Design review of the part built by this model. Coordinates are the model's own, in mm. Face numbers are marked on the shaded views. A direction names the side the tool comes from. Give positions to 0.01 mm unless a question says otherwise; leave off trailing zeros. Loops run counter-clockwise (first coordinate to the right, second up) from the corner with the lowest first, then second, coordinate; pieces in that order, holes last. Notation, with made-up numbers: (66, 23) -> (95, 23) arc R34 ccw to (95, 57) -> close; hole circle Ø8 at (45, 44). An arc over 180 degrees is marked (long way). Use a Markdown table: item, result. Add a question column.
1. Add section B-B (y = 27). State the section outline as (x, z) points, and give its area (4 significant figures).
2. Add section C-C (x = 7). State the section outline as (y, z) points, and give its area (3 significant figures).
3. Add section A-A (z = 5). State the section outline as (x, y) points.
4. For the marked faces 1 and 2, list the 3-axis set-ups (+Z, -Z, +X, -X, +Y, -Y) from which the entire face can be reached by the end or side of a thin tool; tool diameter is ignored.
5. To check wall thickness, follow line 1 (X direction, y = 59, z = 18.5); line 2 (Y direction, x = 26.5, z = 19.25). State the ranges of each line that lie inside material, in increasing order.
6. Draft analysis for pull direction X (two halves, no side actions). For the marked faces 3, 4, 5 and 6, state which applies: pulls with the +X half, pulls with the -X half, needs draft (parallel to the pull), parting line crosses it, or undercut.
7. For pin 1 Ø8 at (x, z) = (72.5, 22.5) entering from -Y, flat-tipped, find the tip position at first contact; note if it passes through.
```python
from build123d import *

# Parameters (mm, degrees)
F0_W     = 110
F0_H     = 110
F0_W_2   = 106
F0_H_2   = 106
F1_DEPTH = 25
F2_W     = 106
F2_H     = 106
F3_DEPTH = 1.5
F4_W     = 25
F4_H     = 25
F5_DEPTH = 25
F6_R     = 26.255837
F7_DEPTH = 1.5
F9_DEPTH = 25


with BuildPart() as f1:
    # F0 (on Top) → F1 (new body)
    with BuildSketch(Plane.XY):
        with Locations((55, 55)):
            Rectangle(F0_W, F0_H)
        with Locations((55, 55)):
            Rectangle(F0_W_2, F0_H_2, mode=Mode.SUBTRACT)
    extrude(amount=F1_DEPTH)

    # F2 (on Top) → F3 (join)
    with BuildSketch(Plane.XY):
        with Locations((55, 55)):
            Rectangle(F2_W, F2_H)
    extrude(amount=F3_DEPTH)

    # F4 (on Top) → F5 (cut)
    with BuildSketch(Plane.XY):
        with Locations((23.550745, 87.610851)):
            Rectangle(F4_W, F4_H)
        with Locations((23.550745, 55.610851)):
            Rectangle(F4_W, F4_H)
        with Locations((23.550745, 23.610851)):
            Rectangle(F4_W, F4_H)
        with Locations((55.550745, 87.610851)):
            Rectangle(F4_W, F4_H)
        with Locations((55.550745, 55.610851)):
            Rectangle(F4_W, F4_H)
        with Locations((55.550745, 23.610851)):
            Rectangle(F4_W, F4_H)
        with Locations((87.550745, 87.610851)):
            Rectangle(F4_W, F4_H)
        with Locations((87.550745, 55.610851)):
            Rectangle(F4_W, F4_H)
        with Locations((87.550745, 23.610851)):
            Rectangle(F4_W, F4_H)
    extrude(amount=F5_DEPTH, mode=Mode.SUBTRACT)

    # F6 (on face) → F7 (join, through all)
    with BuildSketch(Plane.XY.offset(1.5)):
        with Locations((55.742927, 79.293631)):
            Circle(F6_R)
    extrude(amount=-F7_DEPTH)

    # F8 (on face) → F9 (cut)
    with BuildSketch(Plane.XZ):
        with BuildLine():
            Line((100.912742, 28.472882), (10.870284, 28.621467))
            ThreePointArc((10.870284, 28.621467), (55.864304, 12.058173), (100.912742, 28.472882))
        make_face()
    extrude(amount=-F9_DEPTH, mode=Mode.SUBTRACT)


solid = f1.part
```
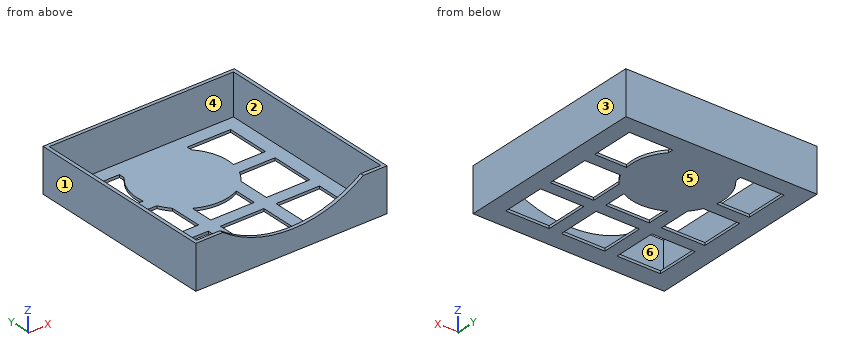
Taken from the geometry:
| question | item | result |
|---|---|---|
| 1 | outline | (0, 0) -> (11.05, 0) -> (11.05, 1.5) -> (2, 1.5) -> (2, 25) -> (0, 25) -> close; (36.05, 0) -> (43.05, 0) -> (43.05, 1.5) -> (36.05, 1.5) -> close; (68.05, 0) -> (75.05, 0) -> (75.05, 1.5) -> (68.05, 1.5) -> close; (100.05, 0) -> (110, 0) -> (110, 25) -> (108, 25) -> (108, 1.5) -> (100.05, 1.5) -> close |
| 1 | area | 146.5 mm^2 |
| 2 | outline | (0, 0) -> (110, 0) -> (110, 25) -> (108, 25) -> (108, 1.5) -> (2, 1.5) -> (2, 25) -> (0, 25) -> close |
| 2 | area | 259 mm^2 |
| 3 | outline | (0, 0) -> (110, 0) -> (110, 110) -> (0, 110) -> close; hole (2, 2) -> (108, 2) -> (108, 108) -> (2, 108) -> close |
| 4 | face 1 | +Z, -Z, -X, +Y, -Y |
| 4 | face 2 | +Z |
| 5 | line 1 | x = 0 to 2, 108 to 110 |
| 5 | line 2 | y = 108 to 110 |
| 6 | face 3 | pulls with the +X half |
| 6 | face 4 | undercut |
| 6 | face 5 | needs draft |
| 6 | face 6 | undercut |
| 7 | pin 1 | stops at y = 108 |
